The listing builds one solid part. Answer for the finished solid, in the listing's coordinates (mm). A direction names the side the tool comes from. Round coordinates to 2 decimals unless told otherwise and drop trailing zeros. Write each loop counter-clockwise with the first axis right and the second up, starting at its lowest first coordinate (ties: lowest second). Pieces come first, ordered by that corner, then holes.
from build123d import *

# Parameters (mm, degrees)
BOSS_EXTRUDE1_DEPTH = 51.31
CUT_EXTRUDE1_DEPTH  = 169.903952009
EXTRUDE_THIN1_START = -51.31
EXTRUDE_THIN1_DEPTH = 102.62


with BuildPart() as part:
    # Sketch1 → Boss-Extrude1 (new, symmetric)
    with BuildSketch(Plane.XY):
        with BuildLine():
            Line((59.876515773, 19.086695264), (57.402885491, -4.903230804))
            ThreePointArc((57.402885491, -4.903230804), (54.121767552, -11.36639665), (47.356152322, -13.9673))
            Line((47.356152322, -13.9673), (42.356152322, -13.9673))
            Line((42.356152322, -13.9673), (42.356152322, -17.293867679))
            Line((42.356152322, -17.293867679), (128.611229128, -17.293867679))
            ThreePointArc((128.611229128, -17.293867679), (131.335936638, -15.549243714), (130.891584134, -12.344513672))
            Line((130.891584134, -12.344513672), (102.990355006, 20.294354008))
            ThreePointArc((102.990355006, 20.294354008), (102.114192176, 20.996083615), (101.041429063, 21.326636258))
            Line((101.041429063, 21.326636258), (58.969893766, 26.003172338))
            ThreePointArc((58.969893766, 26.003172338), (59.828073734, 22.598004621), (59.876515773, 19.086695264))
        make_face()
    extrude(amount=BOSS_EXTRUDE1_DEPTH, both=True)

    # Sketch2 → Cut-Extrude1 (cut, through all)
    with BuildSketch(Plane.XY.offset(51.31)):
        with BuildLine():
            Line((65.02802496, 20.298975288), (62.376515773, -5.416067836))
            ThreePointArc((62.376515773, -5.416067836), (61.55413792, -9.00803973), (59.886234411, -12.293867679))
            Line((59.886234411, -12.293867679), (124.270366416, -12.293867679))
            Line((124.270366416, -12.293867679), (99.70340547, 16.444571904))
            Line((99.70340547, 16.444571904), (65.02802496, 20.298975288))
        make_face()
    extrude(amount=-CUT_EXTRUDE1_DEPTH, mode=Mode.SUBTRACT)

    # Sketch3 → Extrude-Thin1 (add)
    with BuildSketch(Plane.XY.offset(EXTRUDE_THIN1_START)):
        Polygon((99.70340547, 16.444571904), (76.337464228, -12.293867679), (80.216979633, -15.448128325), (103.582920875, 13.290311258), align=None)
        Polygon((124.270366416, -12.293867679), (88.020434849, 2.075352112), (86.177943711, -2.572790141), (122.427875278, -16.942009933), align=None)
        Polygon((65.02802496, 20.298975288), (85.881897007, -0.554896759), (62.877757, -0.554896759), (59.886234411, -0.554896759), (59.886234411, -5.554896759), (62.877757, -5.554896759), (97.952964819, -5.554896759), (68.563558866, 23.834509194), align=None)
    extrude(amount=EXTRUDE_THIN1_DEPTH)


solid = part.part
1. For a pull along X with two mould halves and no side action, classify faces 1 (the face through (75.309, 10.018, -0.718)), 2 (the face through (80.3, 23.632, 0.718)), 3 (the face through (72, -5.555, -1)), 4 (the face through (54.198, -11.296, 0.718)) as released by +X, released by -X, zero draft, split by the parting line, or undercut.
Geometry says:
face 1: undercut
face 2: released by +X
face 3: undercut
face 4: released by -X
2. Given pin 1 (8 mm diameter, centred on x = 67, z = 4, fed in from +Y); pin 2 (5 mm diameter, centred on y = 10, z = -12.5, fed in from -X); pin 3 (10 mm diameter, centred on x = 85.5, z = -38.5, fed in from +Y); pin 4 (6 mm diameter, centred on x = 51.5, y = -4.5, fed in from -Z), each flat-ended and moving along its own axis, determine where each tip first touches the part or whether it passes through.
Geometry says:
pin 1: stops at y = 25.56
pin 2: stops at x = 58.68
pin 3: stops at y = 23.61
pin 4: passes through
3. Section B-B on y = 9.5 is taken. Determine the outline of the cut face in (x, z), plus the area to 3 significant figures.
Geometry says:
outline: (58.89, -51.31) - (63.91, -51.31) - (63.91, 51.31) - (58.89, 51.31) - close; (75.83, -51.31) - (82.9, -51.31) - (82.9, 51.31) - (75.83, 51.31) - close; (94.06, -51.31) - (100.5, -51.31) - (100.5, 51.31) - (94.06, 51.31) - close; (105.64, -51.31) - (112.22, -51.31) - (112.22, 51.31) - (105.64, 51.31) - close
area: 2,580 mm2
4. Section D-D on y = -2 is taken. Determine the outline of the cut face in (x, z), plus the area to 3 significant figures.
Geometry says:
outline: (57.7, -51.31) - (98.3, -51.31) - (98.3, 51.31) - (57.7, 51.31) - close; (115.47, -51.31) - (122.05, -51.31) - (122.05, 51.31) - (115.47, 51.31) - close
area: 4,840 mm2
5. Straight lines are drawn through the part: line 1 along Y through (x, z) = (82.5, 29); line 2 along X through (y, z) = (4, 14.5); line 3 along X through (y, z) = (2.5, 30). For each, find the intervals that lie inside material, in ascending order.
Geometry says:
line 1: y = -17.29 to -0.55, 2.83 to 9.9, 18.36 to 23.39
line 2: x = 58.32 to 63.35, 81.33 to 88.4, 89.59 to 96.03, 110.34 to 116.92
line 3: x = 58.17 to 63.19, 82.83 to 94.81, 111.62 to 118.2
6. A tool of negligible diameter and unlimited length cuts with its end or side. For faces 5 (the face through (79.115, -8.877, -0.718)), 6 (the face through (85, -17.294, 1)), from which of +Z, -Z, +X, -X, +Y, -Y can it reach the whole face along a straight path? Write none if from no direction.
Geometry says:
face 5: +Z, -Z
face 6: +Z, -Z, +X, -X, -Y
7. Section C-C on x = 67.5 is taken. Determine the outline of the cut face in (y, z) (3 decimals).
Geometry says:
outline: (-17.294, -51.31) - (-12.294, -51.31) - (-12.294, 51.31) - (-17.294, 51.31) - close; (-5.555, -51.31) - (-0.555, -51.31) - (-0.555, 51.31) - (-5.555, 51.31) - close; (17.827, -51.31) - (25.055, -51.31) - (25.055, 51.31) - (17.827, 51.31) - close
8. Section A-A on z = 21.5 is taken. Determine the outline of the cut face in (x, y) (3 decimals), plus the area to 3 significant figures.
Geometry says:
outline: (42.356, -17.294) - (128.611, -17.294) arc R3 ccw to (130.892, -12.345) - (102.99, 20.294) arc R3 ccw to (101.041, 21.327) - (58.97, 26.003) arc R15.1 cw to (59.877, 19.087) - (57.403, -4.903) arc R10.1 cw to (47.356, -13.967) - (42.356, -13.967) - close; hole (59.886, -12.294) - (76.337, -12.294) - (81.817, -5.555) - (62.362, -5.555) arc R15.1 cw to start; hole (62.878, -0.555) - (85.882, -0.555) - (65.028, 20.299) - close; hole (72.983, 19.415) - (89.053, 3.345) - (99.703, 16.445) - close; hole (82.782, -12.294) - (110.702, -12.294) - (93.701, -5.555) - (88.261, -5.555) - close; hole (92.894, 0.144) - (124.27, -12.294) - (103.006, 12.581) - close
area: 1,570 mm2
